The model under review builds one solid part; all positions refer to its coordinate system, in mm. A direction names the side the tool comes from. Coordinates: 2 decimals unless noted, no trailing zeros. Loops run counter-clockwise (first coordinate to the right, second up) from the corner with the lowest first, then second, coordinate; pieces in that order, holes last. Notation, with made-up numbers: M -26.5,-38.75 L 25.5,-38.75 A35 cw 25.5,-4.75 Z; hole C 50.5,24 d9. An arc over 180 degrees is marked long. Use one line per item in the form item = value.
```python
from build123d import *

# Parameters (mm, degrees)
F0_R        = 60.565035
F0_R_2      = 50
F1_DEPTH    = 109
F1_FACE_R   = 60.565035
F1_FACE_R_2 = 50
F2_DEPTH    = 25
F3_W        = 148.240149
F3_H        = 161.59083
F4_DEPTH    = 38.407663


with BuildPart() as f1:
    # F0 (on Top) → F1 (new body)
    with BuildSketch(Plane.XY):
        with Locations((-166.333571, 45.535278)):
            Circle(F0_R)
        with Locations((-166.333571, 45.535278)):
            Circle(F0_R_2, mode=Mode.SUBTRACT)
    extrude(amount=F1_DEPTH)

    # F1_face (on face) + F0 (on Top) → F2 (join)
    with BuildSketch(Plane(origin=(-166.333571, 45.535278, 0), x_dir=(1, 0, 0), z_dir=(0, 0, -1))):
        Circle(F1_FACE_R)
        Circle(F1_FACE_R_2, mode=Mode.SUBTRACT)
    with BuildSketch(Plane.XY):
        with Locations((-166.333571, 45.535278)):
            Circle(F0_R)
        with Locations((-166.333571, 45.535278)):
            Circle(F0_R_2, mode=Mode.SUBTRACT)
    extrude(amount=F2_DEPTH)

    # F3 (on Top) → F4 (join)
    with BuildSketch(Plane.XY):
        with Locations((-162.065908, 49.431123)):
            Rectangle(F3_W, F3_H)
    extrude(amount=-F4_DEPTH)


solid = f1.part
```
1. Add section C-C (z = 90.5). State the section outline as (x, y) points.
Response values:
outline = C -166.33,45.54 d121.13; hole C -166.33,45.54 d100
2. The part is to be moulded in two halves that separate along Y. For faces 1 (the face through (-236.186, 48, -19)), 2 (the face through (-120.15, 64.69, 55.26)), 3 (the face through (-226.84, 42.87, 55.26)), say which applies: pulls with the +Y half, pulls with the -Y half, needs draft (parallel to the pull), parting line crosses it, or undercut.
Response values:
face_1 = needs draft
face_2 = undercut
face_3 = parting line crosses it
3. Machinability: for faces 4 (the face through (-147, 104, 0)), 5 (the face through (-163, -31.364, -19)), which of the approach directions +Z, -Z, +X, -X, +Y, -Y give a long, thin tool a straight path to every point of the face, cutting with its end or side? Answer none if there is none.
Response values:
face_4 = +Z
face_5 = +Z, -Z, +X, -X, -Y
4. Add section B-B (x = -169.5). State the section outline as (y, z) points.
Response values:
outline = M -31.36,-38.41 L 130.23,-38.41 L 130.23,0 L 106.02,0 L 106.02,109 L 95.43,109 L 95.43,0 L -4.36,0 L -4.36,109 L -14.95,109 L -14.95,0 L -31.36,0 Z
5. Add section D-D (y = -10). State the section outline as (x, z) points.
Response values:
outline = M -236.19,-38.41 L -87.95,-38.41 L -87.95,0 L -142.17,0 L -142.17,109 L -190.5,109 L -190.5,0 L -236.19,0 Z
6. Add section A-A (y = 58.5). State the section outline as (x, z) points, then the cut area to 3 significant figures.
Response values:
outline = M -236.19,-38.41 L -87.95,-38.41 L -87.95,0 L -107.17,0 L -107.17,109 L -118.04,109 L -118.04,0 L -214.62,0 L -214.62,109 L -225.49,109 L -225.49,0 L -236.19,0 Z
area = 8,060 mm^2
7. Wall thickness on line 1 along X through (y, z) = (47, 1); line 2 along Z through (x, y) = (-229.5, 71); line 3 along Y through (x, z) = (-157, 80.5): over which ranges is each line inside the solid? List them lowest first. Write a range as from..to.
Response values:
line_1 = -226.88..-216.31, -116.36..-105.79
line_2 = -38.41..0
line_3 = -14.31..-3.59, 94.66..105.38
8. Insertion check: P1, Ø3, axis at y = 13, z = 29, coming from the +X side; P2, Ø12, axis at y = 91, z = 72, coming from the -X side; P3, Ø12, axis at y = -10.5, z = 59.5, coming from the +X side. Each pin has a flat end and moves straight along its axis. Give the tip position at first contact, or say it passes through.
Response values:
P1 = -114.32
P2 = -212.28
P3 = -132.21
